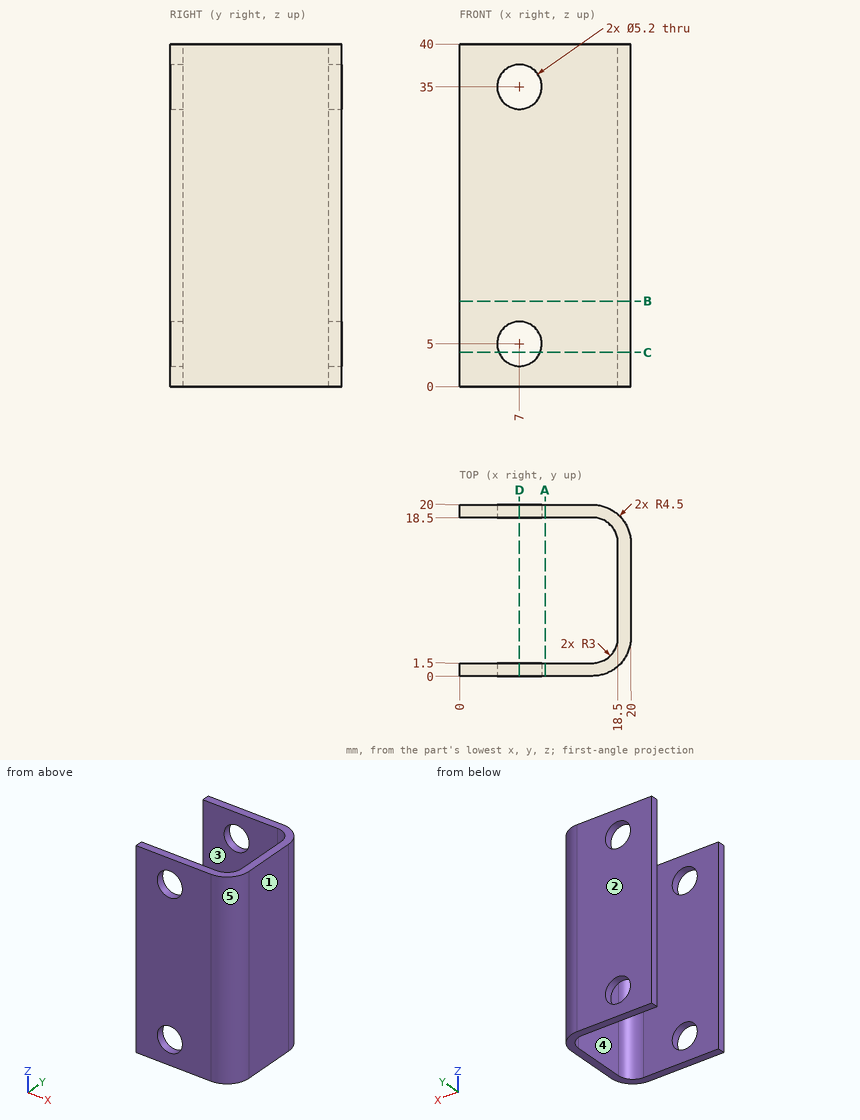
Geometry: see drawing. Coordinates: mm, zero at the bounding-box minimum. A direction names the side the tool comes from. Round coordinates to 2 decimals unless told otherwise and drop trailing zeros. Write each loop counter-clockwise with the first axis right and the second up, starting at its lowest first coordinate (ties: lowest second). Pieces come first, ordered by that corner, then holes.
1) Ray query, L1, parallel to Y at x = 13.5, z = 5; L2, parallel to X at y = 14.75, z = 27.5; L3, parallel to X at y = 0.5, z = 35. Return the intervals inside material, ascending.
2) Cut plane B-B (z = 10). Return the cut outline in (x, y).
3) Draft query along Y for the marked faces 1, 2 and 3. Return one class per face: pulls with the +Y half, pulls with the -Y half, needs draft (parallel to the pull), parting line crosses it, or undercut.
4) Cut plane C-C (z = 4). Return the cut outline in (x, y).
5) Cut plane A-A (x = 10). Return the cut outline in (y, z).
6) Cut plane D-D (x = 7). Return the cut outline in (y, z), then the cut area to 3 significant figures.
7) Contact query for flat-ended pins moving along their axis: P1, Ø9, axis at y = 11.5, z = 15.5, coming from the -X side; P2, Ø4, axis at x = 7, z = 35, coming from the -Y side; P3, Ø3, axis at y = 5, z = 11, coming from the -X side. Output: stop coordinate, or through.
8) Reachability of the marked faces 4 and 5 from +Z, -Z, +X, -X, +Y, -Y: full face, straight path, thin tool, end or side. Return the list, or none.
Geometry says:
1. L1: y = 0 to 1.5, 18.5 to 20
1. L2: x = 18.5 to 20
1. L3: x = 0 to 4.4, 9.6 to 17.56
2. outline: (0, 0) - (15.5, 0) arc R4.5 ccw to (20, 4.5) - (20, 15.5) arc R4.5 ccw to (15.5, 20) - (0, 20) - (0, 18.5) - (15.5, 18.5) arc R3 cw to (18.5, 15.5) - (18.5, 4.5) arc R3 cw to (15.5, 1.5) - (0, 1.5) - close
3. face 1: needs draft
3. face 2: pulls with the +Y half
3. face 3: undercut
4. outline: (0, 0) - (4.6, 0) - (4.6, 1.5) - (0, 1.5) - close; (0, 18.5) - (4.6, 18.5) - (4.6, 20) - (0, 20) - close; (9.4, 0) - (15.5, 0) arc R4.5 ccw to (20, 4.5) - (20, 15.5) arc R4.5 ccw to (15.5, 20) - (9.4, 20) - (9.4, 18.5) - (15.5, 18.5) arc R3 cw to (18.5, 15.5) - (18.5, 4.5) arc R3 cw to (15.5, 1.5) - (9.4, 1.5) - close
5. outline: (0, 0) - (1.5, 0) - (1.5, 40) - (0, 40) - close; (18.5, 0) - (20, 0) - (20, 40) - (18.5, 40) - close
6. outline: (0, 0) - (1.5, 0) - (1.5, 2.4) - (0, 2.4) - close; (0, 7.6) - (1.5, 7.6) - (1.5, 32.4) - (0, 32.4) - close; (0, 37.6) - (1.5, 37.6) - (1.5, 40) - (0, 40) - close; (18.5, 0) - (20, 0) - (20, 2.4) - (18.5, 2.4) - close; (18.5, 7.6) - (20, 7.6) - (20, 32.4) - (18.5, 32.4) - close; (18.5, 37.6) - (20, 37.6) - (20, 40) - (18.5, 40) - close
6. area: 88.8 mm2
7. P1: stops at x = 18.46
7. P2: passes through
7. P3: stops at x = 18.33
8. face 4: +Z, -Z, -X
8. face 5: +Z, -Z, +X, -Y
